The listing builds one solid part. Answer for the finished solid, in the listing's coordinates (mm). A direction names the side the tool comes from. Round coordinates to 2 decimals unless told otherwise and drop trailing zeros. Write each loop counter-clockwise with the first axis right and the second up, starting at its lowest first coordinate (ties: lowest second). Pieces come first, ordered by that corner, then holes.
Item 1: Each of these flat-tipped pins is pushed along its axis until it touches: pin 1 (12.5 mm diameter, centred on y = -33.5, z = 17, fed in from -X); pin 2 (1 mm diameter, centred on y = 14, z = 7, fed in from -X); pin 3 (1 mm diameter, centred on x = -44, z = 1.5, fed in from +Y); pin 4 (2 mm diameter, centred on x = -37.5, y = -20, fed in from -Z). Where does it stop, or does it pass through?
Item 2: Find section B-B on y = -55.5. Give the vertices of the cut face in (x, z) (3 decimals), then the cut area to 3 significant figures.
Item 3: Find section A-A on y = 9. Give the vertices of the cut face in (x, z) (3 decimals).
Item 4: Find section C-C on x = -54. Give the vertices of the cut face in (y, z) (3 decimals), then the cut area to 3 significant figures.
Item 5: Find section D-D on z = 15. Give the number of separate pieces and of enclosed holes in the cut face, then the cut area to 3 significant figures.
Item 6: Find the intervals of material crossed by probe 1 along X at (y, z) = (39.5, 47.5); probe 2 along X at (y, z) = (5, 44.5); probe 3 along Y at (x, z) = (-33, 15.5), in increasing order.
Item 7: For a pull along X with two mould halves and no side action, classify faces 4 (the face through (9, -19, 50.8)), 5 (the face through (-55.15, -18.96, 25.04)), 6 (the face through (40.819, 37, 25)), 7 (the face through (32.84, -57.24, 25.04)) as +X half, -X half, draft (parallel to the pull), parting line (faces both ways), or undercut.
Item 8: A tool of negligible diameter and unlimited length cuts with its end or side. For faces 1 (the face through (-43.994, -38, 25)), 2 (the face through (-31.276, -54.476, 26.654)), 3 (the face through (43.994, 38, 25)), from which of +Z, -Z, +X, -X, +Y, -Y can it reach the whole face along a straight path? Write none if from no direction.
```python
from build123d import *

# Parameters (mm, degrees)
F1_DEPTH = 50.8
F2_DEPTH = 3.175


with BuildPart() as f1:
    # F0 (on Top) → F1 (new body)
    with BuildSketch(Plane.XY):
        Polygon((-42.419291, 22.643037), (-40.819091, 23.566913), (-43.994091, 25.4), (-65.991136, 12.7), (-65.991136, -12.7), (-43.994091, -25.4), (-40.819091, -23.566913), (-42.419291, -22.643037), (-46.8187, -20.103037), (-62.816136, -10.866913), (-62.816136, 10.866913), (-46.8187, 20.103037), align=None)
        Polygon((-1.6002, 48.057702), (0, 47.133826), (0, 50.8), (-21.997045, 63.5), (-43.994091, 50.8), (-43.994091, 25.4), (-40.819091, 23.566913), (-40.819091, 25.414665), (-40.819091, 30.494665), (-40.819091, 48.966913), (-21.997045, 59.833826), (-5.999609, 50.597702), align=None)
        Polygon((0, 50.8), (0, 47.133826), (1.6002, 48.057702), (5.999609, 50.597702), (21.997045, 59.833826), (40.819091, 48.966913), (40.819091, 30.494665), (40.819091, 28.646913), (40.819091, 25.414665), (40.819091, 23.566913), (43.994091, 25.4), (43.994091, 50.8), (21.997045, 63.5), align=None)
        Polygon((42.419291, -22.643037), (40.819091, -23.566913), (43.994091, -25.4), (65.991136, -12.7), (65.991136, 12.7), (43.994091, 25.4), (40.819091, 23.566913), (42.419291, 22.643037), (46.8187, 20.103037), (62.816136, 10.866913), (62.816136, -10.866913), (46.8187, -20.103037), align=None)
        Polygon((43.994091, -25.4), (40.819091, -23.566913), (40.819091, -25.414665), (40.819091, -30.494665), (40.819091, -48.966913), (21.997045, -59.833826), (5.999609, -50.597702), (1.6002, -48.057702), (0, -47.133826), (0, -50.8), (21.997045, -63.5), (43.994091, -50.8), align=None)
        Polygon((-40.819091, -25.4), (-40.819091, -23.566913), (-43.994091, -25.4), (-43.994091, -50.8), (-21.997045, -63.5), (0, -50.8), (0, -47.133826), (-1.6002, -48.057702), (-4.399409, -49.673826), (-21.997045, -59.833826), (-40.819091, -48.966913), (-40.819091, -30.48), (-40.819091, -25.414665), align=None)
        Polygon((-21.997045, -12.7), (-21.997045, 12.7), (-40.819091, 23.566913), (-42.419291, 22.643037), (-38.019881, 20.103037), (-23.597245, 11.776124), (-23.597245, -11.776124), (-38.019881, -20.103037), (-42.419291, -22.643037), (-40.819091, -23.566913), align=None)
        Polygon((-21.997045, 12.7), (0, 25.4), (0, 47.133826), (-1.6002, 48.057702), (-1.6002, 42.977702), (-1.6002, 26.323876), (-21.997045, 14.547752), (-36.419681, 22.874665), (-40.819091, 25.414665), (-40.819091, 23.566913), align=None)
        Polygon((21.997045, 12.7), (0, 25.4), (0, 23.552248), (4.399409, 21.012248), (20.396845, 11.776124), (20.396845, -11.776124), (21.997045, -12.7), align=None)
        Polygon((0, -25.4), (-21.997045, -12.7), (-40.819091, -23.566913), (-40.819091, -25.4), (-36.413345, -22.871006), (-21.997045, -14.547752), (-1.6002, -26.323876), (-1.6002, -42.977702), (-1.6002, -48.057702), (0, -47.133826), align=None)
        Polygon((21.997045, -14.547752), (21.997045, -12.7), (0, -25.4), (1.6002, -26.323876), align=None)
        Polygon((0, 47.133826), (0, 25.4), (21.997045, 12.7), (36.419681, 21.026913), (40.819091, 23.566913), (40.819091, 25.414665), (36.419681, 22.874665), (21.997045, 14.547752), (1.6002, 26.323876), (1.6002, 42.977702), (1.6002, 48.057702), align=None)
        Polygon((36.419681, 21.026913), (21.997045, 12.7), (21.997045, -12.7), (40.819091, -23.566913), (42.419291, -22.643037), (38.019881, -20.103037), (23.597245, -11.776124), (23.597245, 11.776124), (38.019881, 20.103037), (42.419291, 22.643037), (40.819091, 23.566913), align=None)
        Polygon((0, 23.552248), (0, 25.4), (-21.997045, 12.7), (-20.396845, 11.776124), (-4.399409, 21.012248), align=None)
        Polygon((40.819091, -23.566913), (21.997045, -12.7), (21.997045, -14.547752), (36.419681, -22.874665), (40.819091, -25.414665), align=None)
        Polygon((1.6002, -26.323876), (0, -25.4), (0, -47.133826), (1.6002, -48.057702), (1.6002, -42.977702), align=None)
        Polygon((-20.396845, 11.776124), (-21.997045, 12.7), (-21.997045, -12.7), (0, -25.4), (0, -23.552248), (-4.399409, -21.012248), (-20.396845, -11.776124), align=None)
        Polygon((0, -25.4), (21.997045, -12.7), (20.396845, -11.776124), (4.399409, -21.012248), (0, -23.552248), align=None)
    extrude(amount=F1_DEPTH)

    # F0 (on Top) → F2 (join)
    with BuildSketch(Plane.XY):
        Polygon((-1.6002, 42.977702), (-5.999609, 50.597702), (-21.997045, 59.833826), (-40.819091, 48.966913), (-40.819091, 30.494665), (-36.419681, 22.874665), (-21.997045, 14.547752), (-1.6002, 26.323876), align=None)
        Polygon((-38.019881, 20.103037), (-46.8187, 20.103037), (-62.816136, 10.866913), (-62.816136, -10.866913), (-46.8187, -20.103037), (-38.019881, -20.103037), (-23.597245, -11.776124), (-23.597245, 11.776124), align=None)
        Polygon((-4.399409, 21.012248), (-20.396845, 11.776124), (-20.396845, -11.776124), (-4.399409, -21.012248), (4.399409, -21.012248), (20.396845, -11.776124), (20.396845, 11.776124), (4.399409, 21.012248), align=None)
        Polygon((21.997045, 59.833826), (5.999609, 50.597702), (1.6002, 42.977702), (1.6002, 26.323876), (21.997045, 14.547752), (36.419681, 22.874665), (40.819091, 30.494665), (40.819091, 48.966913), align=None)
        Polygon((38.019881, -20.103037), (46.8187, -20.103037), (62.816136, -10.866913), (62.816136, 10.866913), (46.8187, 20.103037), (38.019881, 20.103037), (23.597245, 11.776124), (23.597245, -11.776124), align=None)
        Polygon((36.419681, -22.874665), (21.997045, -14.547752), (1.6002, -26.323876), (1.6002, -42.977702), (5.999609, -50.597702), (21.997045, -59.833826), (40.819091, -48.966913), (40.819091, -30.494665), align=None)
        Polygon((-21.997045, -14.547752), (-36.413345, -22.871006), (-40.819091, -30.48), (-40.819091, -48.966913), (-21.997045, -59.833826), (-4.399409, -49.673826), (-1.6002, -42.977702), (-1.6002, -26.323876), align=None)
        Polygon((0, 23.552248), (0, 25.4), (-21.997045, 12.7), (-20.396845, 11.776124), (-4.399409, 21.012248), align=None)
    extrude(amount=F2_DEPTH)


solid = f1.part
```
Check values:
1. pin 1: stops at x = -43.99
1. pin 2: stops at x = -64.61
1. pin 3: stops at y = 51.09
1. pin 4: stops at z = 0
2. outline: (-35.853, 0) - (-8.141, 0) - (-8.141, 50.8) - (-14.491, 50.8) - (-14.491, 3.175) - (-29.503, 3.175) - (-29.503, 50.8) - (-35.853, 50.8) - close; (8.141, 0) - (35.853, 0) - (35.853, 50.8) - (29.503, 50.8) - (29.503, 3.175) - (14.491, 3.175) - (14.491, 50.8) - (8.141, 50.8) - close
2. area: 1,390 mm2
3. outline: (-65.991, 0) - (65.991, 0) - (65.991, 50.8) - (62.816, 50.8) - (62.816, 3.175) - (23.597, 3.175) - (23.597, 50.8) - (20.397, 50.8) - (20.397, 3.175) - (-20.397, 3.175) - (-20.397, 50.8) - (-23.597, 50.8) - (-23.597, 3.175) - (-62.816, 3.175) - (-62.816, 50.8) - (-65.991, 50.8) - close
4. outline: (-19.623, 0) - (19.623, 0) - (19.623, 50.8) - (15.957, 50.8) - (15.957, 3.175) - (-15.957, 3.175) - (-15.957, 50.8) - (-19.623, 50.8) - close
4. area: 474 mm2
5. separate pieces: 1
5. enclosed holes: 7
5. area: 2,300 mm2
6. probe 1: x = -43.99 to -40.82, -1.6 to 1.6, 40.82 to 43.99
6. probe 2: x = -65.99 to -62.82, -23.6 to -20.4, 20.4 to 23.6, 62.82 to 65.99
6. probe 3: y = -57.15 to -53.48, -20.9 to -17.2, 17.2 to 20.9, 53.48 to 57.15
7. face 4: draft
7. face 5: -X half
7. face 6: undercut
7. face 7: +X half
8. face 1: +Z, -Z, -X, -Y
8. face 2: +Z
8. face 3: +Z, -Z, +X, +Y
